Geometry check sheet. Reference: the model listing, model coordinates, mm. Give positions to 0.01 mm unless a question says otherwise; leave off trailing zeros. Write each loop counter-clockwise with the first axis right and the second up, starting at its lowest first coordinate (ties: lowest second). Pieces come first, ordered by that corner, then holes. Notation, with made-up numbers: (84, 31.5) - (142, 31.5) arc R24 ccw to (142, 46.5) - close; hole circle Ø8 at (-20, -17). An arc over 180 degrees is marked (long way). One line per question, with ' | ' between items. Start each with the question number.
Q1. Section check A-A on x = 30. Record the boundary of the cut face in (y, z).
Q2. Thickness scan on L1, parallel to X at y = 1.25, z = -7; L2, parallel to X at y = 3, z = -22; L3, parallel to Z at x = 48.5, y = 1. Record the ranges inside material, lowest first. Write a range as [from, to].
Q3. Section check B-B on z = -1. Record the boundary of the cut face in (x, y).
Q4. Section check D-D on z = 12.5. Record the boundary of the cut face in (x, y), and give its area (3 significant figures).
Q5. Section check C-C on y = 4. Count the separate pieces of the cut face and the enclosed holes in it, and give its area (3 significant figures).
Q6. Gauge pin test, flat end, axial feed: P1, Ø2, axis at y = 5.5, z = -6.5, coming from the -X side. Record the tip position at first contact, or that the pin passes through.
```python
from build123d import *

# Parameters (mm, degrees)
SKETCH1_W                   = 254
SKETCH1_H                   = 50.8
BOSS_EXTRUDE1_DEPTH         = 6.35
F_1_4_0_25_DIAMETER_HOLE1_D = 6.35
FILLET1_R                   = 25.4
SKETCH4_W                   = 40.64
SKETCH4_H                   = 25.4
CUT_EXTRUDE1_DEPTH          = 25.4


with BuildPart() as part:
    # Sketch1 → Boss-Extrude1 (new body)
    with BuildSketch(Plane(origin=(0, 0, 0), x_dir=(1, 0, 0), z_dir=(0, 1, 0))):
        with Locations((92.878696742, 9.930827068)):
            Rectangle(SKETCH1_W, SKETCH1_H)
    extrude(amount=BOSS_EXTRUDE1_DEPTH)

    # 1/4 (0.25) Diameter Hole1 (through all)
    with Locations(Plane(origin=(0, 6.35, 0), x_dir=(1, 0, 0), z_dir=(0, 1, 0))):
        with Locations((-21.421303258, 9.930827068), (181.778696742, 9.930827068)):
            Hole(F_1_4_0_25_DIAMETER_HOLE1_D / 2)

    # Fillet1
    fillet1_edges = [part.edges().sort_by_distance(p)[0] for p in [
        (-34.121303258, 3.175, 15.469172932),
        (-34.121303258, 3.175, -35.330827068),
    ]]
    fillet(fillet1_edges, radius=FILLET1_R - 0.0001)  # a hair under: the kernel refuses the full size

    # Sketch4 → Cut-Extrude1 (cut)
    with BuildSketch(Plane(origin=(0, 6.35, 0), x_dir=(1, 0, 0), z_dir=(0, 1, 0))):
        with Locations((36.998696742, 9.930827068)):
            Rectangle(SKETCH4_W, SKETCH4_H)
    extrude(amount=-CUT_EXTRUDE1_DEPTH, mode=Mode.SUBTRACT)


solid = part.part
```
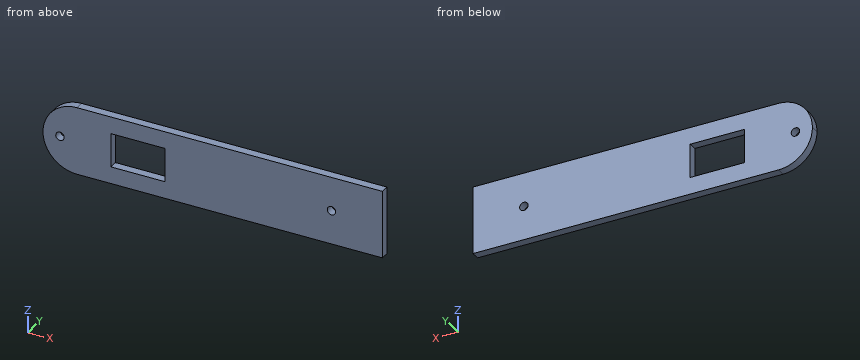
Working result:
1) outline: (0, -35.33) - (6.35, -35.33) - (6.35, -22.63) - (0, -22.63) - close; (0, 2.77) - (6.35, 2.77) - (6.35, 15.47) - (0, 15.47) - close
2) L1: x = [-33.95, -22.64], [-20.2, 16.68], [57.32, 180.56], [183, 219.88] | L2: x = [-31.07, 16.68], [57.32, 219.88] | L3: z = [-35.33, -22.63], [2.77, 15.47]
3) outline: (-32.5, 0) - (16.68, 0) - (16.68, 6.35) - (-32.5, 6.35) - close; (57.32, 0) - (219.88, 0) - (219.88, 6.35) - (57.32, 6.35) - close
4) outline: (-20.64, 0) - (219.88, 0) - (219.88, 6.35) - (-20.64, 6.35) - close | area: 1,530 mm2
5) separate pieces: 1 | enclosed holes: 3 | area: 11,500 mm2
6) P1: stops at x = -34
